Build history of the part. All positions in model axes, mm. Face numbers are marked on the shaded views. A direction names the side the tool comes from. Give positions to 0.01 mm unless a question says otherwise; leave off trailing zeros. Loops run counter-clockwise (first coordinate to the right, second up) from the corner with the lowest first, then second, coordinate; pieces in that order, holes last. Notation, with made-up numbers: M -4.5,40 L 17.5,40 A25 cw 17.5,76 Z; hole C 88,57.25 d9. An arc over 180 degrees is marked long. Put each result on its own line as item: value.
```python
from build123d import *

# Parameters (mm, degrees)
SKETCH1_R           = 7.5
SKETCH1_R_2         = 10
BOSS_EXTRUDE1_DEPTH = 10


with BuildPart() as part:
    # Sketch1 → Boss-Extrude1 (new, symmetric)
    with BuildSketch(Plane.XY):
        with BuildLine():
            ThreePointArc((0, 20), (-20, 0), (0, -20))
            Line((0, -20), (10, -20))
            ThreePointArc((10, -20), (13.535533906, -21.464466094), (15, -25))
            Line((15, -25), (15, -45))
            ThreePointArc((15, -45), (19.393398282, -55.606601718), (30, -60))
            ThreePointArc((30, -60), (40.606601718, -64.393398282), (45, -75))
            ThreePointArc((45, -75), (49.393398282, -85.606601718), (60, -90))
            Line((60, -90), (100, -90))
            Line((100, -90), (105, -85))
            Line((105, -85), (105, 15))
            Line((105, 15), (100, 20))
            Line((100, 20), (82.320508076, 20))
            ThreePointArc((82.320508076, 20), (77.990381057, 22.5), (77.990381057, 27.5))
            ThreePointArc((77.990381057, 27.5), (68.882285677, 49.488887394), (50, 35))
            ThreePointArc((50, 35), (48.984060464, 31.978864085), (46.349095113, 30.185444737))
            Line((46.349095113, 30.185444737), (10, 20))
            Line((10, 20), (0, 20))
        make_face()
        with Locations((30, -45)):
            Circle(SKETCH1_R, mode=Mode.SUBTRACT)
        with Locations((60, -75)):
            Circle(SKETCH1_R, mode=Mode.SUBTRACT)
        with BuildLine():
            ThreePointArc((62.185835481, -50.618244574), (54.053641254, -50.618244574), (54.053641254, -42.486050347))
            Line((54.053641254, -42.486050347), (75.26684469, -21.272846911))
            ThreePointArc((75.26684469, -21.272846911), (83.399038917, -21.272846911), (83.399038917, -29.405041138))
            Line((83.399038917, -29.405041138), (62.185835481, -50.618244574))
        make_face(mode=Mode.SUBTRACT)
        Circle(SKETCH1_R_2, mode=Mode.SUBTRACT)
        with Locations((65, 35)):
            Circle(SKETCH1_R, mode=Mode.SUBTRACT)
    extrude(amount=BOSS_EXTRUDE1_DEPTH, both=True)


solid = part.part
```
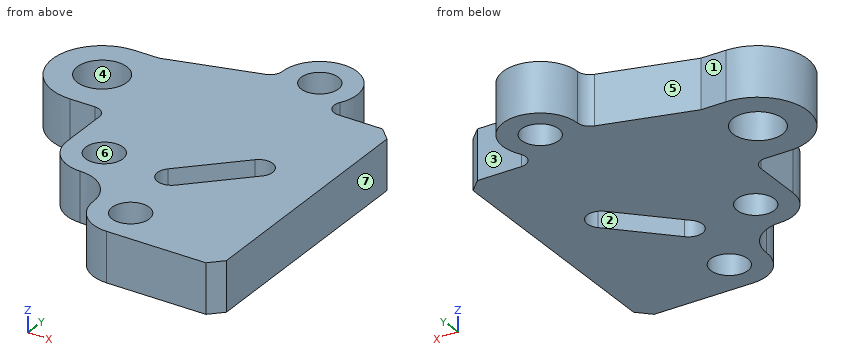
Q1. Slice it at B-B (x = 32.5). List the corners of the cut face in (y, z).
Here are the results:
outline: M -60.21,-10 L -52.07,-10 L -52.07,10 L -60.21,10 Z; M -37.93,-10 L 26.3,-10 L 26.3,10 L -37.93,10 Z
Q2. Tool access for the marked faces 1, 2 and 3: list every direction of +Z, -Z, +X, -X, +Y, -Y with a clear straight run to the whole face (end or side of a thin tool).
Here are the results:
face 1: +Z, -Z, -X, +Y
face 2: +Z, -Z
face 3: +Z, -Z, +X, +Y
Q3. Slice it at A-A (y = -23). List the corners of the cut face in (x, z).
Here are the results:
outline: M 14.58,-10 L 73.54,-10 L 73.54,10 L 14.58,10 Z; M 84.59,-10 L 105,-10 L 105,10 L 84.59,10 Z
Q4. Drop flat-ended pins along their axis: pin 1 Ø2 at (y, z) = (3, 7) entering from -X; pin 2 Ø12 at (x, y) = (0, 0) entering from +Z; pin 3 Ø9 at (x, z) = (95, 1) entering from +Y; pin 4 Ø6 at (y, z) = (-30.5, 0.5) entering from -X. Give the stop position or say it passes through.
Here are the results:
pin 1: x = -19.9
pin 2: through
pin 3: y = 20
pin 4: x = 15
Q5. Probe line 1 (X direction, y = -44, z = -5); line 2 (X direction, y = -49.5, z = -6.25); line 3 (Y direction, x = 65, z = 4.75). List the from-to ranges inside material, lowest first. Write a range as from..to.
Here are the results:
line 1: 15..22.57, 37.43..52.97, 68.8..105
line 2: 15.69..24, 36..53.18, 63.3..105
line 3: -90..-80.59, -69.41..-47.8, -31.54..27.5, 42.5..50
Q6. Mould opens along Y. For the marked faces 4, 5, 6 and 7 say: pulls with the +Y half, pulls with the -Y half, needs draft (parallel to the pull), parting line crosses it, or undercut.
Here are the results:
face 4: undercut
face 5: pulls with the +Y half
face 6: undercut
face 7: needs draft
Q7. Slice it at C-C (z = 2.25). List the corners of the cut face in (x, y), and give its area (3 significant figures).
Here are the results:
outline: M 0,-20 L 10,-20 A5 cw 15,-25 L 15,-45 A15 ccw 30,-60 A15 cw 45,-75 A15 ccw 60,-90 L 100,-90 L 105,-85 L 105,15 L 100,20 L 82.32,20 A5 cw 77.99,27.5 A15 ccw long 50,35 A5 cw 46.35,30.19 L 10,20 L 0,20 A20 ccw Z; hole C 0,0 d20; hole C 30,-45 d15; hole C 60,-75 d15; hole M 54.05,-42.49 A5.75 ccw 62.19,-50.62 L 83.4,-29.41 A5.75 ccw 75.27,-21.27 Z; hole C 65,35 d15
area: 9,880 mm²
